Design review of the part built by this model. Coordinates are the model's own, in mm. Coordinates: 2 decimals unless noted, no trailing zeros.
Q1. For P1, Ø1, axis at y = -85, z = 5, coming from the +X side; P2, Ø2, axis at x = -102, z = 3.5, coming from the -Y side; P3, Ø3, axis at x = -97, z = 5, coming from the +Y side, all flat-tipped, find the tip position at first contact; note any pin that passes through.
Q2. Add section A-A on x = 10. Give the number of separate pieces and of enclosed holes in the cut face, and give its area (3 significant figures).
Q3. Wall thickness on probe 1 along X at (y, z) = (-45, 1.75); probe 2 along X at (y, z) = (130.5, 3.75); probe 3 along Y at (x, z) = (-22.5, 2): over which ranges is each line inside the solid? List them lowest first.
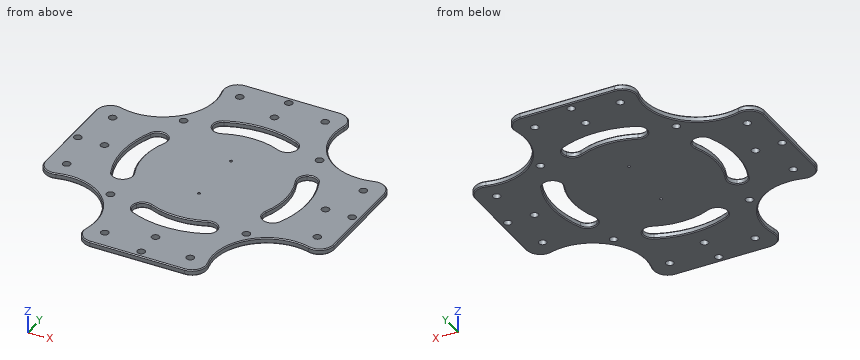
```python
from build123d import *

# Parameters (mm, degrees)
IZIM1_R                     = 4
Y_KSEKLIK_EKSTR_ZYON1_DEPTH = 6
RADYUS1_R                   = 5
IZIM2_R                     = 4
KES_EKSTR_ZYON1_DEPTH       = 10
DAIRESEL_KAPLAMA1_COUNT     = 4
SKETCH1_W                   = 170.605519564
SKETCH1_H                   = 25.837050878
CUT_EXTRUDE1_DEPTH          = 10
CIRPATTERN1_COUNT           = 4
FILLET1_R                   = 50
CUT_EXTRUDE2_DEPTH          = 10
CUT_EXTRUDE3_DEPTH          = 10
FILLET2_R                   = 10
CIRPATTERN3_COUNT           = 4
FILLET2_OF_CIRPATTERN3_R    = 10
CIRPATTERN2_COUNT           = 4
CHAMFER1_SIZE               = 1
SKETCH4_R                   = 1.5
CUT_EXTRUDE4_DEPTH          = 10


with BuildPart() as part:
    # Çizim1 → Yükseklik-Ekstrüzyon1 (new body)
    with BuildSketch(Plane.XY):
        with BuildLine():
            Line((-150.466489, 42), (-150.466489, -42))
            Line((-150.466489, -42), (-159.565033764, -42))
            ThreePointArc((-159.565033764, -42), (-116.672618896, -116.672618896), (-42, -159.565033764))
            Line((-42, -159.565033764), (-42, -150.466489))
            Line((-42, -150.466489), (42, -150.466489))
            Line((42, -150.466489), (42, -159.565033764))
            ThreePointArc((42, -159.565033764), (116.672618896, -116.672618896), (159.565033764, -42))
            Line((159.565033764, -42), (150.466489, -42))
            Line((150.466489, -42), (150.466489, 42))
            Line((150.466489, 42), (159.565033764, 42))
            ThreePointArc((159.565033764, 42), (116.672618896, 116.672618896), (42, 159.565033764))
            Line((42, 159.565033764), (42, 150.466489))
            Line((42, 150.466489), (-42, 150.466489))
            Line((-42, 150.466489), (-42, 159.565033764))
            ThreePointArc((-42, 159.565033764), (-116.672618896, 116.672618896), (-159.565033764, 42))
            Line((-159.565033764, 42), (-150.466489, 42))
        make_face()
        with Locations((0, 115)):
            Circle(IZIM1_R, mode=Mode.SUBTRACT)
        with Locations((115, 0)):
            Circle(IZIM1_R, mode=Mode.SUBTRACT)
        with Locations((0, -115)):
            Circle(IZIM1_R, mode=Mode.SUBTRACT)
        with Locations((-115, 0)):
            Circle(IZIM1_R, mode=Mode.SUBTRACT)
        with Locations((-70.710678119, 70.710678119)):
            Circle(IZIM1_R, mode=Mode.SUBTRACT)
        with Locations((70.710678119, 70.710678119)):
            Circle(IZIM1_R, mode=Mode.SUBTRACT)
        with Locations((70.710678119, -70.710678119)):
            Circle(IZIM1_R, mode=Mode.SUBTRACT)
        with Locations((-70.710678119, -70.710678119)):
            Circle(IZIM1_R, mode=Mode.SUBTRACT)
    extrude(amount=Y_KSEKLIK_EKSTR_ZYON1_DEPTH)

    # Radyus1
    radyus1_edges = [part.edges().sort_by_distance(p)[0] for p in [
        (159.565033764, -42, 3),
        (42, -159.565033764, 3),
        (-42, -159.565033764, 3),
        (-159.565033764, -42, 3),
        (-159.565033764, 42, 3),
        (-42, 159.565033764, 3),
        (42, 159.565033764, 3),
        (159.565033764, 42, 3),
    ]]
    fillet(radyus1_edges, radius=RADYUS1_R)

    # Çizim2 → Kes-Ekstrüzyon1 (cut)
    with BuildSketch(Plane.XY.offset(6)):
        with Locations((-130.466488641, -44.496935975)):
            Circle(IZIM2_R)
        with Locations((-142.73324432, -0.000677265)):
            Circle(IZIM2_R)
        with Locations((-130.466488641, 44.495581446)):
            Circle(IZIM2_R)
    kes_ekstr_zyon1 = extrude(amount=-KES_EKSTR_ZYON1_DEPTH, mode=Mode.SUBTRACT)

    # Dairesel Kaplama1: Kes-Ekstrüzyon1 ×4 about axis
    dairesel_kaplama1_axis = Axis((0, 0, 0), (0, 0, 1))
    for i in range(1, DAIRESEL_KAPLAMA1_COUNT):
        add(kes_ekstr_zyon1.rotate(dairesel_kaplama1_axis, i * 360 / DAIRESEL_KAPLAMA1_COUNT), mode=Mode.SUBTRACT)

    # Sketch1 → Cut-Extrude1 (cut)
    with BuildSketch(Plane(origin=(0, 0, 0), x_dir=(-1, 0, 0), z_dir=(0, 0, -1))):
        with Locations((0, 163.385014439)):
            Rectangle(SKETCH1_W, SKETCH1_H)
    cut_extrude1 = extrude(amount=-CUT_EXTRUDE1_DEPTH, mode=Mode.SUBTRACT)

    # CirPattern1: Cut-Extrude1 ×4 about axis
    cirpattern1_axis = Axis((0, 0, 0), (0, 0, 1))
    for i in range(1, CIRPATTERN1_COUNT):
        add(cut_extrude1.rotate(cirpattern1_axis, i * 360 / CIRPATTERN1_COUNT), mode=Mode.SUBTRACT)

    # Fillet1
    fillet1_edges = [part.edges().sort_by_distance(p)[0] for p in [
        (67.711414754, 150.466489, 3),
        (-67.711414754, 150.466489, 3),
        (-150.466489, 67.711414754, 3),
        (-150.466489, -67.711414754, 3),
        (-67.711414754, -150.466489, 3),
        (67.711414754, -150.466489, 3),
        (150.466489, 67.711414754, 3),
        (150.466489, -67.711414754, 3),
    ]]
    fillet(fillet1_edges, radius=FILLET1_R)

    # Sketch2 → Cut-Extrude2 (cut)
    with BuildSketch(Plane(origin=(0, 0, 0), x_dir=(-1, 0, 0), z_dir=(0, 0, -1))):
        with BuildLine():
            Line((-49.24272607, 150.466489), (-49.24272607, 163.848097422))
            Line((-49.24272607, 163.848097422), (-162.900639376, 163.848097422))
            Line((-162.900639376, 163.848097422), (-162.900639376, 49.24272607))
            Line((-162.900639376, 49.24272607), (-150.466489, 49.24272607))
            ThreePointArc((-150.466489, 49.24272607), (-144.538179355, 61.188622189), (-131.439231121, 63.691988818))
            ThreePointArc((-131.439231121, 63.691988818), (-77.781745931, 77.781745931), (-63.691988818, 131.439231121))
            ThreePointArc((-63.691988818, 131.439231121), (-61.188622189, 144.538179355), (-49.24272607, 150.466489))
        make_face()
    cut_extrude2 = extrude(amount=-CUT_EXTRUDE2_DEPTH, mode=Mode.SUBTRACT)

    # Sketch3 → Cut-Extrude3 (cut)
    with BuildSketch(Plane(origin=(0, 0, 0), x_dir=(-1, 0, 0), z_dir=(0, 0, -1))):
        with BuildLine():
            Line((-64.951905284, 37.5), (-82.27241336, 47.5))
            ThreePointArc((-82.27241336, 47.5), (-95, 0), (-82.27241336, -47.5))
            Line((-82.27241336, -47.5), (-64.951905284, -37.5))
            ThreePointArc((-64.951905284, -37.5), (-75, 0), (-64.951905284, 37.5))
        make_face()
    cut_extrude3 = extrude(amount=-CUT_EXTRUDE3_DEPTH, mode=Mode.SUBTRACT)

    # Fillet2
    fillet2_edges = [part.edges().sort_by_distance(p)[0] for p in [
        (82.27241336, -47.5, 3),
        (64.951905284, -37.5, 3),
        (64.951905284, 37.5, 3),
        (82.27241336, 47.5, 3),
    ]]
    fillet(fillet2_edges, radius=FILLET2_R - 0.0001)  # a hair under: the kernel refuses the full size

    # CirPattern3: Cut-Extrude3 ×4 about axis
    cirpattern3_axis = Axis((0, 0, 0), (0, 0, 1))
    for i in range(1, CIRPATTERN3_COUNT):
        add(cut_extrude3.rotate(cirpattern3_axis, i * 360 / CIRPATTERN3_COUNT), mode=Mode.SUBTRACT)

    # Fillet2 of CirPattern3
    fillet2_of_cirpattern3_edges = [part.edges().sort_by_distance(p)[0] for p in [
        (47.5, 82.27241336, 3),
        (37.5, 64.951905284, 3),
        (-37.5, 64.951905284, 3),
        (-47.5, 82.27241336, 3),
        (-82.27241336, 47.5, 3),
        (-64.951905284, 37.5, 3),
        (-64.951905284, -37.5, 3),
        (-82.27241336, -47.5, 3),
        (-47.5, -82.27241336, 3),
        (-37.5, -64.951905284, 3),
        (37.5, -64.951905284, 3),
        (47.5, -82.27241336, 3),
    ]]
    fillet(fillet2_of_cirpattern3_edges, radius=FILLET2_OF_CIRPATTERN3_R - 0.0001)  # a hair under: the kernel refuses the full size

    # CirPattern2: Cut-Extrude2 ×4 about axis
    cirpattern2_axis = Axis((0, 0, 0), (0, 0, 1))
    for i in range(1, CIRPATTERN2_COUNT):
        add(cut_extrude2.rotate(cirpattern2_axis, i * 360 / CIRPATTERN2_COUNT), mode=Mode.SUBTRACT)

    # Chamfer1
    chamfer1_edges = [part.edges().sort_by_distance(p)[0] for p in [
        (0, 150.466489, 0),
        (0, 150.466489, 6),
        (61.188622189, 144.538179355, 6),
        (77.781745931, 77.781745931, 6),
        (144.538179355, 61.188622189, 6),
        (144.538179355, 61.188622189, 0),
        (77.781745931, 77.781745931, 0),
        (61.188622189, 144.538179355, 0),
        (95, 0, 6),
        (95, 0, 0),
        (75, 0, 6),
        (75, 0, 0),
        (81.25384104, -43.03461599, 0),
        (81.25384104, -43.03461599, 6),
        (68.610961465, -36.697482988, 0),
        (68.610961465, -36.697482988, 6),
        (68.610961465, 36.697482988, 0),
        (68.610961465, 36.697482988, 6),
        (81.25384104, 43.03461599, 0),
        (81.25384104, 43.03461599, 6),
        (0, 95, 6),
        (0, 95, 0),
        (0, 75, 6),
        (0, 75, 0),
        (43.03461599, 81.25384104, 0),
        (43.03461599, 81.25384104, 6),
        (36.697482988, 68.610961465, 0),
        (36.697482988, 68.610961465, 6),
        (-36.697482988, 68.610961465, 0),
        (-36.697482988, 68.610961465, 6),
        (-43.03461599, 81.25384104, 0),
        (-43.03461599, 81.25384104, 6),
        (-95, 0, 6),
        (-95, 0, 0),
        (-75, 0, 6),
        (-75, 0, 0),
        (-81.25384104, 43.03461599, 0),
        (-81.25384104, 43.03461599, 6),
        (-68.610961465, 36.697482988, 0),
        (-68.610961465, 36.697482988, 6),
        (-68.610961465, -36.697482988, 0),
        (-68.610961465, -36.697482988, 6),
        (-81.25384104, -43.03461599, 0),
        (-81.25384104, -43.03461599, 6),
        (0, -95, 6),
        (0, -95, 0),
        (0, -75, 6),
        (0, -75, 0),
        (-43.03461599, -81.25384104, 0),
        (-43.03461599, -81.25384104, 6),
        (-36.697482988, -68.610961465, 0),
        (-36.697482988, -68.610961465, 6),
        (36.697482988, -68.610961465, 0),
        (36.697482988, -68.610961465, 6),
        (43.03461599, -81.25384104, 0),
        (43.03461599, -81.25384104, 6),
        (150.466489, 0, 0),
        (150.466489, 0, 6),
        (0, -150.466489, 0),
        (0, -150.466489, 6),
        (-150.466489, 0, 0),
        (-150.466489, 0, 6),
        (-77.781745931, 77.781745931, 6),
        (-61.188622189, 144.538179355, 6),
        (-144.538179355, 61.188622189, 6),
        (-61.188622189, 144.538179355, 0),
        (-77.781745931, 77.781745931, 0),
        (-144.538179355, 61.188622189, 0),
        (-77.781745931, -77.781745931, 6),
        (-144.538179355, -61.188622189, 6),
        (-61.188622189, -144.538179355, 6),
        (-144.538179355, -61.188622189, 0),
        (-77.781745931, -77.781745931, 0),
        (-61.188622189, -144.538179355, 0),
        (77.781745931, -77.781745931, 6),
        (61.188622189, -144.538179355, 6),
        (144.538179355, -61.188622189, 6),
        (61.188622189, -144.538179355, 0),
        (77.781745931, -77.781745931, 0),
        (144.538179355, -61.188622189, 0),
    ]]
    chamfer(chamfer1_edges, length=CHAMFER1_SIZE)

    # Sketch4 → Cut-Extrude4 (cut)
    with BuildSketch(Plane.XY.offset(6)):
        with Locations((0, 31)):
            Circle(SKETCH4_R)
        with Locations((0, -31)):
            Circle(SKETCH4_R)
    extrude(amount=-CUT_EXTRUDE4_DEPTH, mode=Mode.SUBTRACT)


solid = part.part
```
Entries:
1. P1: stops at x = 72.06
1. P2: stops at y = -63.95
1. P3: stops at y = 65.91
2. separate pieces: 3
2. enclosed holes: 0
2. area: 1,560 mm2
3. probe 1: x = -150.47 to -134.43, -126.5 to 126.5, 134.43 to 150.47
3. probe 2: x = -63.44 to -48.5, -40.5 to 40.5, 48.5 to 63.44
3. probe 3: y = -150.47 to -92.3, -71.55 to 71.55, 92.3 to 150.47
